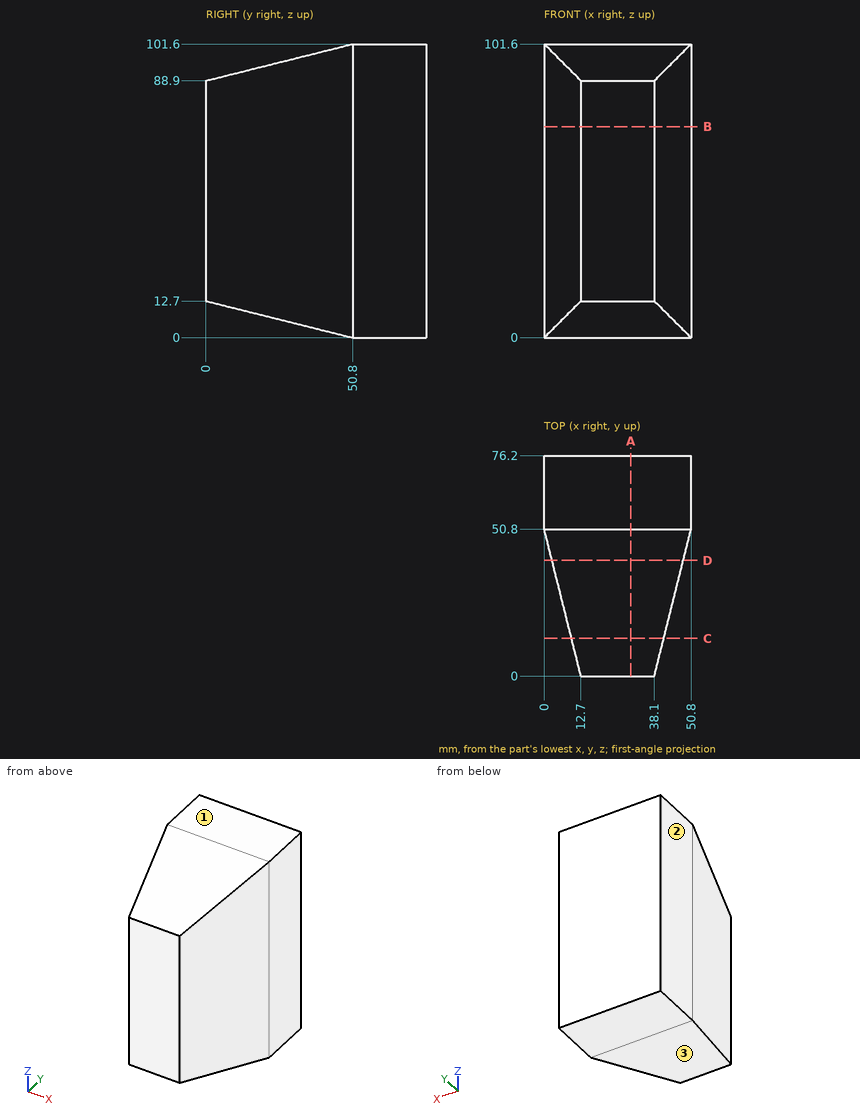
Answer from the drawing. Dimensions are ordinates in mm from the lowest x, y and z of the part. Give positions to 0.01 mm unless a question says otherwise; leave off trailing zeros. Loops run counter-clockwise (first coordinate to the right, second up) from the corner with the lowest first, then second, coordinate; pieces in that order, holes last. Notation, with made-up numbers: (25, -38.5) -> (59, -38.5) arc R21 ccw to (59, -14.5) -> close; hole circle Ø6 at (88, 69.25). An arc over 180 degrees is marked (long way). Answer as CSV lines item,"result".
Item 1: Find section A-A on x = 30. Give the vertices of the cut face in (y, z), plus the area to 3 significant figures.
Returned:
outline,"(0, 12.7) -> (50.8, 0) -> (76.2, 0) -> (76.2, 101.6) -> (50.8, 101.6) -> (0, 88.9) -> close"
area,"7,100 mm²"
Item 2: Each of these flat-tipped pins is pushed along its axis until it touches: pin 1 (1.5 mm diameter, centred on x = 24.5, y = 30.5, fed in from -Z); pin 2 (2 mm diameter, centred on y = 14, z = 18.5, fed in from -X); pin 3 (2 mm diameter, centred on y = 16, z = 13, fed in from +X). Where does it stop, or does it pass through?
Returned:
pin 1,"stops at z = 4.89"
pin 2,"stops at x = 8.95"
pin 3,"stops at x = 42.35"
Item 3: Find section B-B on z = 73. Give the vertices of the cut face in (x, y).
Returned:
outline,"(0, 50.8) -> (12.7, 0) -> (38.1, 0) -> (50.8, 50.8) -> (50.8, 76.2) -> (0, 76.2) -> close"
Item 4: Find section D-D on y = 40. Give the vertices of the cut face in (x, z), plus the area to 3 significant figures.
Returned:
outline,"(2.7, 2.7) -> (48.1, 2.7) -> (48.1, 98.9) -> (2.7, 98.9) -> close"
area,"4,370 mm²"
Item 5: Determine the mould class of the marked faces 1, 2 and 3 for opening direction Z: +Z half, -Z half, draft (parallel to the pull), parting line (faces both ways), or undercut.
Returned:
face 1,"+Z half"
face 2,"draft"
face 3,"-Z half"
Item 6: Consider line 1 (Z direction, x = 14.5, y = 5); line 2 (X direction, y = 25.5, z = 24) (3 decimals); line 3 (Z direction, x = 38.5, y = 12). Determine where each line is inside the solid, lowest interval first. Write a range as [from, to].
Returned:
line 1,"z = [11.45, 90.15]"
line 2,"x = [6.325, 44.475]"
line 3,"z = [9.7, 91.9]"
Item 7: Find section C-C on y = 13. Give the vertices of the cut face in (x, z).
Returned:
outline,"(9.45, 9.45) -> (41.35, 9.45) -> (41.35, 92.15) -> (9.45, 92.15) -> close"
